For this review, take the finished solid that the model builds, in its own axes (mm). Coordinates: 2 decimals unless noted, no trailing zeros. Loops run counter-clockwise (first coordinate to the right, second up) from the corner with the lowest first, then second, coordinate; pieces in that order, holes last. Notation, with made-up numbers: (43.5, 76) -> (70.5, 76) arc R25 ccw to (70.5, 115) -> close; hole circle Ø7 at (55, 37.25). An arc over 180 degrees is marked (long way). Answer in a Markdown table with one row per item.
Autodesk Inventor part; units mm, degrees
ref_plane "YZ Plane" through (0, 0, 0) normal (1, 0, 0) x (0, 1, 0)
ref_plane "XZ Plane" through (0, 0, 0) normal (0, 1, 0) x (-1, 0, 0)
ref_plane "XY Plane" through (0, 0, 0) normal (0, 0, 1) x (1, 0, 0)
sketch "Эскиз1" plane through (0, 0, 0) normal (0, 1, 0) x (-1, 0, 0)
  line L0 (0, 0) -> (388, 0)
  line L1 (388, 0) -> (388, -508)
  line L2 (388, -508) -> (0, -508)
  line L3 (0, -508) -> (0, 0)
  dimension "d0" = 388
  dimension "d1" = 508
extrude "Выдавливание1" add sketch "Эскиз1" along normal blind 4
sketch "Эскиз2" plane through (0, 4, 0) normal (0, 1, 0) x (1, 0, 0)
  line L0 (-388, 508) -> (-388, 0)
  line L1 (-388, 149) -> (-257, 149)
  line L2 (-257, 149) -> (-257, 275)
  line L3 (-257, 275) -> (-388, 275)
  line L4 (-388, 275) -> (-388, 149)
  line L5 (0, 0) -> (-5, 0)
  line L6 (-388, 0) -> (0, 0)
  line L7 (-388, 0) -> (-384, 0)
  line L8 (-384, 0) -> (-384, 4)
  line L9 (-384, 4) -> (-388, 4)
  line L10 (-388, 4) -> (-388, 0)
  line L11 (0, 508) -> (-388, 508)
  line L12 (-388, 508) -> (-384, 508)
  line L13 (-384, 508) -> (-384, 504)
  line L14 (-384, 504) -> (-388, 504)
  line L15 (-388, 504) -> (-388, 508)
  point P0 (-388, 275)
  dimension "d4" = 126
  dimension "d5" = 131
  dimension "d13" = 149
  dimension "d14" = 4
  dimension "d15" = 4
  dimension "d16" = 4
  dimension "d17" = 4
extrude "Выдавливание3" cut sketch "Эскиз2" against normal blind 10
properties part number "MountingWallSide2"
Item 1: Insertion check: pin 1 (4 mm diameter, centred on x = -88.5, z = -304.5, fed in from -Y); pin 2 (1.2 mm diameter, centred on y = 2, z = -184.5, fed in from -X). Each pin has a flat end and moves straight along its axis. Give the tip position at first contact, or say it passes through.
Worked answers:
| item | result |
|---|---|
| pin 1 | y = 0 |
| pin 2 | x = -257 |
Item 2: Take a section at B-B, the plane y = 0.85. State the section outline as (x, z) points, and give its area (3 significant figures).
Worked answers:
| item | result |
|---|---|
| outline | (-388, -504) -> (-384, -504) -> (-384, -508) -> (0, -508) -> (0, 0) -> (-384, 0) -> (-384, -4) -> (-388, -4) -> (-388, -149) -> (-257, -149) -> (-257, -275) -> (-388, -275) -> close |
| area | 181,000 mm² |
Item 3: For L1, parallel to Z at x = -333, y = 1.7; L2, parallel to X at y = 1.6, z = -258, list the stretches that pass through material, from the lowest coordinate up.
Worked answers:
| item | result |
|---|---|
| L1 | -508 to -275, -149 to 0 |
| L2 | -257 to 0 |
Item 4: Take a section at A-A, the plane x = -273. State the section outline as (y, z) points, and give its area (3 significant figures).
Worked answers:
| item | result |
|---|---|
| outline | (0, -508) -> (4, -508) -> (4, -275) -> (0, -275) -> close; (0, -149) -> (4, -149) -> (4, 0) -> (0, 0) -> close |
| area | 1,530 mm² |
Item 5: Take a section at C-C, the plane z = -198. State the section outline as (x, y) points, and give its area (3 significant figures).
Worked answers:
| item | result |
|---|---|
| outline | (-257, 0) -> (0, 0) -> (0, 4) -> (-257, 4) -> close |
| area | 1,030 mm² |
